Work out the finished part from the listing and answer in its coordinate system (mm). A direction names the side the tool comes from. Coordinates: 2 decimals unless noted, no trailing zeros. Order: outer loops, then holes, each group sorted by start corner. A loop starts at its lowest first (then second) coordinate and runs counter-clockwise, first axis right, second up.
1. Flat-ended cylindrical pins translate along their axes: pin 1 Ø8 at (x, y) = (0, -24) entering from +Z; pin 2 Ø1.7 at (x, y) = (4.5, 8) entering from -Z; pin 3 Ø1 at (x, y) = (-11.5, 14.5) entering from +Z. Find the tip coordinate at first contact, or state that the pin passes through.
2. Determine the mould class of faces 3 (the flat face through (0, 0, 3.545)), 4 (the conical face through (-0.346, -21.366, 7.907)), 5 (the flat face through (15, 0, 6)) for opening direction X: +X half, -X half, draft (parallel to the pull), parting line (faces both ways), or undercut.
3. A tool of negligible diameter and unlimited length cuts with its end or side. For faces 1 (the flat face through (0, -7, 5)), 2 (the cylindrical face through (11.481, 18.385, 9.145)), from which of +Z, -Z, +X, -X, +Y, -Y can it reach the whole face along a straight path? Write none if from no direction.
4. Find the intervals of material crossed by probe 1 along Y at (x, z) = (0, 3.25); probe 2 along Y at (x, z) = (0, 6.25); probe 3 along X at (y, z) = (0, 6.65), in increasing order.
5. The part is cut by section B-B, the plane x = 0. Give the vertices of the cut face in (y, z) (3 decimals).
6. The part is cut by section C-C, the plane y = 0. Give the vertices of the cut face in (x, z) (3 decimals), then the cut area to 3 significant figures.
7. The part is cut by section A-A, the plane z = 2.5. Give the vertices of the cut face in (x, y).
8. The part is cut by section D-D, the plane y = 7. Give the vertices of the cut face in (x, z).
```python
from build123d import *

# Parameters (mm, degrees)
F0_R     = 2.55
F1_DEPTH = 10
F2_W     = 20.1
F2_H     = 5
F3_DEPTH = 30.001
F5_DEPTH = 30
F6_DEPTH = 10
F7_R     = 3
F8_SIZE  = 2.2


# Not quite as in the source:
# - a feature names something its author has since deleted; it is built from what else it names


with BuildPart() as f1:
    # F0 (on Top) → F1 (new body)
    with BuildSketch(Plane.XY):
        with BuildLine():
            Line((-9.7593021288, 27.0148037464), (-15, 10.05))
            Line((-15, 10.05), (-15, -10.05))
            Line((-15, -10.05), (-9.7593021288, -27.0148037464))
            ThreePointArc((-9.7593021288, -27.0148037464), (0, -34.21435361), (9.7593021288, -27.0148037464))
            Line((9.7593021288, -27.0148037464), (15, -10.05))
            Line((15, -10.05), (15, 10.05))
            Line((15, 10.05), (9.7593021288, 27.0148037464))
            ThreePointArc((9.7593021288, 27.0148037464), (0, 34.21435361), (-9.7593021288, 27.0148037464))
        make_face()
        with Locations((-7, 0)):
            Circle(F0_R, mode=Mode.SUBTRACT)
        with Locations((0, 24)):
            Circle(F0_R, mode=Mode.SUBTRACT)
        with Locations((0, -24)):
            Circle(F0_R, mode=Mode.SUBTRACT)
    extrude(amount=F1_DEPTH)

    # F2 (on face) → F3 (cut, through all)
    with BuildSketch(Plane.YZ.offset(15)):
        with Locations((0, 2.5)):
            Rectangle(F2_W, F2_H)
    extrude(amount=-F3_DEPTH, mode=Mode.SUBTRACT)

    # F4 (on face) → F5 (join, through all)
    with BuildSketch(Plane.YZ.offset(15)):
        Polygon((3.05, 3.545), (4.5, 5), (-4.5, 5), (-3.05, 3.545), align=None)
    extrude(amount=-F5_DEPTH)

    # F0 (on Top) → F6 (cut, through all)
    with BuildSketch(Plane.XY):
        with Locations((-7, 0)):
            Circle(F0_R)
    extrude(amount=F6_DEPTH, mode=Mode.SUBTRACT)

    # F7
    f7_edges = [f1.edges().sort_by_distance(p)[0] for p in [
        (-12.379651, 18.532402, 10),
        (12.379651, 18.532402, 10),
        (12.379651, -18.532402, 10),
        (-12.379651, -18.532402, 10),
        (15, 0, 10),
        (-15, 0, 10),
    ]]
    fillet(f7_edges, radius=F7_R)

    # F8
    f8_edges = [f1.edges().sort_by_distance(p)[0] for p in [
        (-2.55, -24, 10),
        (-9.55, 0, 10),
        (-2.55, 24, 10),
    ]]
    chamfer(f8_edges, length=F8_SIZE)


solid = f1.part
```
Geometry says:
1. pin 1: stops at z = 9.25
1. pin 2: stops at z = 5
1. pin 3: stops at z = 9.96
2. face 3: draft
2. face 4: undercut
2. face 5: +X half
3. face 1: -Z, +X, -X
3. face 2: +Z, +X, +Y
4. probe 1: y = -34.21 to -26.55, -21.45 to -10.05, 10.05 to 21.45, 26.55 to 34.21
4. probe 2: y = -34.21 to -26.55, -21.45 to 21.45, 26.55 to 34.21
4. probe 3: x = -15 to -9.55, -4.45 to 15
5. outline: (-34.214, 0) - (-26.55, 0) - (-26.55, 7.8) - (-28.75, 10) - (-31.214, 10) arc R3 ccw to (-34.214, 7) - close; (-21.45, 0) - (-10.05, 0) - (-10.05, 5) - (-4.5, 5) - (-3.05, 3.545) - (3.05, 3.545) - (4.5, 5) - (10.05, 5) - (10.05, 0) - (21.45, 0) - (21.45, 7.8) - (19.25, 10) - (-19.25, 10) - (-21.45, 7.8) - close; (26.55, 0) - (34.214, 0) - (34.214, 7) arc R3 ccw to (31.214, 10) - (28.75, 10) - (26.55, 7.8) - close
6. outline: (-15, 3.545) - (-9.55, 3.545) - (-9.55, 7.8) - (-11.75, 10) - (-12, 10) arc R3 ccw to (-15, 7) - close; (-4.45, 3.545) - (15, 3.545) - (15, 7) arc R3 ccw to (12, 10) - (-2.25, 10) - (-4.45, 7.8) - close
6. area: 152 mm2
7. outline: (-15, -10.05) - (-9.76, -27.01) arc R10.21 ccw to (9.76, -27.01) - (15, -10.05) - close; (-15, 10.05) - (15, 10.05) - (9.76, 27.01) arc R10.21 ccw to (-9.76, 27.01) - close; hole circle Ø5.1 at (0, -24); hole circle Ø5.1 at (0, 24)
8. outline: (-15, 5) - (15, 5) - (15, 7) arc R3 ccw to (12, 10) - (-12, 10) arc R3 ccw to (-15, 7) - close
